Check sheet for the modelled part. Datum: model origin and axes. Units: mm. A direction names the side the tool comes from. Coordinates: 2 decimals unless noted, no trailing zeros. Write each loop counter-clockwise with the first axis right and the second up, starting at its lowest first coordinate (ties: lowest second). Pieces come first, ordered by that corner, then holes. Notation, with made-up numbers: (82.5, 15) -> (88.5, 15) arc R4 cw to (88.5, 22) -> close; hole circle Ø4 at (-39.5, 14.25). An arc over 180 degrees is marked (long way). One line per item, written item: value. Start each with the question number.
1) Sectioned sample at D-D on z = 3.5. Enter the section's corners in (x, y).
2) Sectioned sample at C-C on y = 14. Enter the section's corners in (x, z), plus the area to 3 significant figures.
3) Sectioned sample at A-A on x = 0. Give the number of separate pieces and of enclosed holes in the cut face, plus the area to 3 significant figures.
4) Gauge pin test, flat end, axial feed: P1, Ø1, axis at x = 5.5, z = 6.5, coming from the +Y side. Record the tip position at first contact, or that the pin passes through.
5) Scan lines: line 1 along Y through (x, z) = (5, 12); line 2 along Y through (x, z) = (10.5, 14.25); line 3 along X through (y, z) = (-14.95, 10.16). Record each from-to range of solid material in increasing order. Write a range as [from, to].
6) Set-up check for faces 4 (the cylindrical face through (0.212, 15.609, 11.134)), 5 (the flat face through (-10, 0.238, 12)), 6 (the cylindrical face through (-7.439, 4.167, 14.257)), 7 (the flat face through (0, -11.725, 6)): record each of +Z, -Z, +X, -X, +Y, -Y from which the full face is reachable in a straight line by a thin tool's end or side.
7) Draft check along Y on faces 1 (the flat face through (-0.178, -13.729, 2.576)), 2 (the flat face through (0, 4, 10.16)), 3 (the flat face through (0, -1, 0)). Enter one of: +Y half, -Y half, draft (parallel to the pull), parting line (faces both ways), or undercut.
8) Sectioned sample at B-B on y = -10.5. Enter the section's corners in (x, z).
```python
from build123d import *

# Parameters (mm, degrees)
SKETCH1_W                    = 25.4
SKETCH1_H                    = 33.02
BOSS_EXTRUDE1_DEPTH          = 15.24
SKETCH2_W                    = 13.462
SKETCH2_H                    = 13.462
CUT_EXTRUDE1_DEPTH           = 5.08
SKETCH3_W                    = 11.45304241
SKETCH3_H                    = 5.762537062
CUT_EXTRUDE2_DEPTH           = 26.80944982
CHAMFER1_SIZE                = 5.08
CHAMFER1_SIZE_2              = 5.641911575
F_1_4_CLEARANCE_HOLE1_REACH  = 40.521
F_1_4_CLEARANCE_HOLE1_BORE_R = 3.3782
F_4_CLEARANCE_HOLE1_D        = 3.2639
F_4_CLEARANCE_HOLE1_DEPTH    = 6.102100278
F_4_CLEARANCE_HOLE2_D        = 3.2639
CHAMFER2_SIZE                = 8.89
SKETCH11_W                   = 6.858
SKETCH11_H                   = 2.794
SKETCH11_W_2                 = 2.794
SKETCH11_H_2                 = 6.858
CUT_EXTRUDE3_DEPTH           = 6.0833


with BuildPart() as part:
    # Sketch1 → Boss-Extrude1 (new body)
    with BuildSketch(Plane.XY):
        Rectangle(SKETCH1_W, SKETCH1_H)
    extrude(amount=BOSS_EXTRUDE1_DEPTH)

    # Sketch2 → Cut-Extrude1 (cut)
    with BuildSketch(Plane.XY.offset(15.24)):
        with Locations((0, 3.676899722)):
            Rectangle(SKETCH2_W, SKETCH2_H)
    extrude(amount=-CUT_EXTRUDE1_DEPTH, mode=Mode.SUBTRACT)

    # Sketch3 → Cut-Extrude2 (cut, through all)
    with BuildSketch(Plane.XY.offset(15.24)):
        with Locations((0, -8.844079083)):
            Rectangle(SKETCH3_W, SKETCH3_H)
    extrude(amount=-CUT_EXTRUDE2_DEPTH, mode=Mode.SUBTRACT)

    # Chamfer1
    # the kernel refuses this chamfer: 5.641911575, 5.08 mm, written as the material it takes off along each edge
    with BuildSketch(Plane(origin=(-27.228960176, -16.51, 0), x_dir=(0, -0.03204434000819542, 0.9994864482690293), z_dir=(1, 0, 0))) as chamfer1_piece_1:
        Polygon((CHAMFER1_SIZE * 0.999486448269, -CHAMFER1_SIZE * 0.0320443400082), (-CHAMFER1_SIZE_2 * 0.0320443400101, -CHAMFER1_SIZE_2 * 0.999486448328), (0, 0), align=None)
    extrude(amount=54.457920352, mode=Mode.SUBTRACT)

    # 1/4 Clearance Hole1 bore → 1/4 Clearance Hole1 (cut, up to next)
    with BuildSketch(Plane(origin=(0, -16.51, 0), x_dir=(-1, 0, 0), z_dir=(0, -1, 0)), mode=Mode.PRIVATE) as f_1_4_clearance_hole1_sk1:
        with Locations((0, -10.16)):
            Circle(F_1_4_CLEARANCE_HOLE1_BORE_R)
    f_1_4_clearance_hole1_tool1 = extrude(f_1_4_clearance_hole1_sk1.sketch, amount=-F_1_4_CLEARANCE_HOLE1_REACH, mode=Mode.PRIVATE) & part.part
    add(f_1_4_clearance_hole1_tool1.solids().sort_by_distance((0, -16.51, 10.16))[0], mode=Mode.SUBTRACT)

    # #4 Clearance Hole1
    with Locations(Plane(origin=(0, 16.51, 0), x_dir=(1, 0, 0), z_dir=(0, 1, 0))):
        with Locations((0, -12.752259571)):
            Hole(F_4_CLEARANCE_HOLE1_D / 2, depth=F_4_CLEARANCE_HOLE1_DEPTH)

    # #4 Clearance Hole2 (through all)
    with Locations(Plane(origin=(12.7, 0, 0), x_dir=(0, 0, -1), z_dir=(1, 0, 0))):
        with Locations((-12.7, 3.676899722)):
            Hole(F_4_CLEARANCE_HOLE2_D / 2)

    # Chamfer2
    chamfer2_edges = [part.edges().sort_by_distance(p)[0] for p in [
        (0, 16.51, 0),
    ]]
    chamfer(chamfer2_edges, length=CHAMFER2_SIZE)

    # Sketch11 → Cut-Extrude3 (cut)
    with BuildSketch(Plane.XY.offset(15.24)):
        with Locations((0, 13.335)):
            Rectangle(SKETCH11_W, SKETCH11_H)
        with Locations((9.525, 3.667057181)):
            Rectangle(SKETCH11_W_2, SKETCH11_H_2)
        with Locations((-9.525, 3.667057181)):
            Rectangle(SKETCH11_W_2, SKETCH11_H_2)
    extrude(amount=-CUT_EXTRUDE3_DEPTH, mode=Mode.SUBTRACT)


solid = part.part
```
Answers:
1. outline: (-12.7, -14.76) -> (12.7, -14.76) -> (12.7, 11.12) -> (-12.7, 11.12) -> close; hole (-5.73, -11.73) -> (5.73, -11.73) -> (5.73, -5.96) -> (-5.73, -5.96) -> close
2. outline: (-12.7, 6.38) -> (12.7, 6.38) -> (12.7, 15.24) -> (3.43, 15.24) -> (3.43, 9.16) -> (-3.43, 9.16) -> (-3.43, 15.24) -> (-12.7, 15.24) -> close
2. area: 183 mm2
3. separate pieces: 5
3. enclosed holes: 0
3. area: 233 mm2
4. P1: stops at y = 14.62
5. line 1: y = [-16.51, -11.73], [-5.96, -3.05], [10.41, 16.51]
5. line 2: y = [-16.51, 0.24], [7.1, 16.51]
5. line 3: x = [-12.7, -3.38], [3.38, 12.7]
6. face 4: +Y
6. face 5: +Z
6. face 6: +X, -X
6. face 7: +Z, -Z
7. face 1: -Y half
7. face 2: undercut
7. face 3: draft
8. outline: (-12.7, 0) -> (-5.73, 0) -> (-5.73, 15.24) -> (-12.7, 15.24) -> close; (5.73, 0) -> (12.7, 0) -> (12.7, 15.24) -> (5.73, 15.24) -> close
